Autodesk Inventor part; units mm, degrees
ref_plane "YZ Plane" through (0, 0, 0) normal (1, 0, 0) x (0, 1, 0)
ref_plane "XZ Plane" through (0, 0, 0) normal (0, 1, 0) x (-1, 0, 0)
ref_plane "XY Plane" through (0, 0, 0) normal (0, 0, 1) x (1, 0, 0)
sketch "Boceto1" plane through (0, 0, 0) normal (0, 0, 1) x (1, 0, 0)
  line L0 (254.0457, 0) -> (177.0228, 110)
  line L1 (77.0228, 110) -> (0, 0)
  line L2 (84.5228, 110) -> (84.5228, 55)
  line L3 (84.5228, 55) -> (96.5228, 55)
  line L4 (96.5228, 55) -> (96.5228, 110)
  line L5 (157.5228, 110) -> (157.5228, 55)
  line L6 (157.5228, 55) -> (169.5228, 55)
  line L7 (169.5228, 55) -> (169.5228, 110)
  line L8 (84.5228, 110) -> (77.0228, 110)
  line L9 (177.0228, 110) -> (169.5228, 110)
  line L10 (157.5228, 110) -> (96.5228, 110)
  line L11 (0, 0) -> (40.0401, 0)
  line L12 (40.0401, 0) -> (254.0457, 0)
  dimension "d1" = 100
  dimension "d2" = 110
  dimension "d3" = 61
  dimension "d5" = 12
  dimension "d6" = 7.5
  dimension "d12" = 55
  dimension "d23" = 55
  dimension "d24" = 55
extrude "Extrusión1" add sketch "Boceto1" along normal blind 6
sketch "Boceto3" plane through (0, 0, 6) normal (0, 0, 1) x (1, 0, 0)
  line L0 (0, 0) -> (254.0457, 0)
  line L1 (50, 9) -> (50, 0)
  line L2 (45, 0) -> (45, 9)
  line L3 (43.5, 12) -> (51.5, 12)
  line L4 (51.5, 12) -> (51.5, 9)
  line L5 (43.5, 9) -> (43.5, 12)
  line L6 (51.5, 9) -> (50, 9)
  line L7 (45, 9) -> (43.5, 9)
  line L8 (157.5228, 110) -> (96.5228, 110)
  line L9 (127.0228, 110) -> (127.0228, 0)
  line L10 (204.0457, 9) -> (204.0457, 0)
  line L11 (209.0457, 0) -> (209.0457, 9)
  line L12 (210.5457, 12) -> (202.5457, 12)
  line L13 (202.5457, 12) -> (202.5457, 9)
  line L14 (210.5457, 9) -> (210.5457, 12)
  line L15 (202.5457, 9) -> (204.0457, 9)
  line L16 (209.0457, 9) -> (210.5457, 9)
  line L17 (45, 0) -> (50, 0) construction
  line L18 (204.0457, 0) -> (209.0457, 0) construction
  point P0 (204.0457, 0)
  point P1 (47.5, 12)
  point P2 (47.5, 0)
  point P3 (206.5457, 0)
  dimension "d25" = 5
  dimension "d26" = 8
  dimension "d27" = 12
  dimension "d29" = 45
  dimension "d30" = 3
extrude "Extrusión3" cut sketch "Boceto3" against normal up to next
sketch "Boceto4" plane through (0, 0, 0) normal (0, -1, 0) x (1, 0, 0)
  line L0 (77.0228, 6) -> (0, 6)
  line L1 (77.0228, 0) -> (0, 0)
  line L2 (38.5114, 6) -> (28.5114, 6)
  line L3 (28.5114, 6) -> (28.5114, 0)
  line L4 (28.5114, 0) -> (38.5114, 0)
  line L5 (38.5114, 0) -> (38.5114, 6)
  line L6 (50, 0) -> (204.0457, 0)
  line L7 (56.5114, 6) -> (66.5114, 6)
  line L8 (66.5114, 6) -> (66.5114, 0)
  line L9 (66.5114, 0) -> (56.5114, 0)
  line L10 (56.5114, 0) -> (56.5114, 6)
  line L11 (157.5228, 0) -> (96.5228, 0)
  line L12 (127.0228, 0) -> (127.0228, 6) construction
  line L13 (215.5342, 6) -> (225.5342, 6)
  line L14 (225.5342, 6) -> (225.5342, 0)
  line L15 (225.5342, 0) -> (215.5342, 0)
  line L16 (215.5342, 0) -> (215.5342, 6)
  line L17 (197.5342, 6) -> (187.5342, 6)
  line L18 (187.5342, 6) -> (187.5342, 0)
  line L19 (187.5342, 0) -> (197.5342, 0)
  line L20 (197.5342, 0) -> (197.5342, 6)
  dimension "d33" = 10
  dimension "d34" = 18
  dimension "d35" = 10
extrude "Extrusión4" add sketch "Boceto4" along normal blind 3 contours L8 L1 L10 L0 | L18 L17 L20 L6 | L5 L1 L3 L0 | L13 L14 L15 L16
sketch "Boceto5" plane through (0, 0, 6) normal (0, 0, 1) x (1, 0, 0)
  circle A0 centre (127.0228, 32) radius 2
  line L0 (66.5114, 0) -> (187.5342, 0)
  line L1 (157.5228, 110) -> (96.5228, 110)
  point P0 (0, 0)
  point P1 (127.0228, 110)
  dimension "d39" = 4
  dimension "d40" = 32
extrude "Extrusión5" cut sketch "Boceto5" against normal through all
properties part number "UnionColumnas"
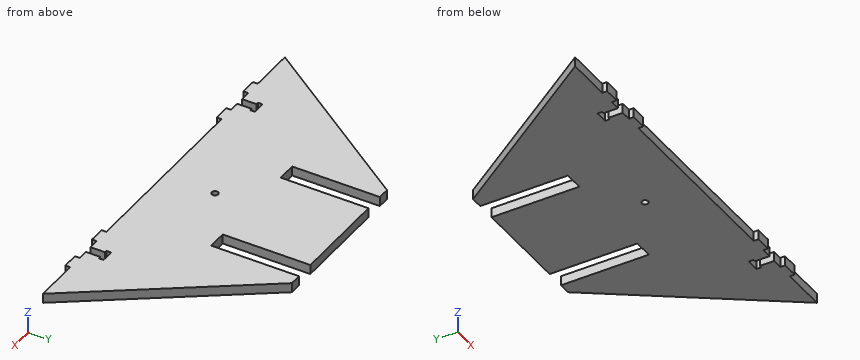
The listing builds one solid part. Answer for the finished solid, in the listing's coordinates (mm). Round coordinates to 2 decimals unless told otherwise and drop trailing zeros. Write each loop counter-clockwise with the first axis right and the second up, starting at its lowest first coordinate (ties: lowest second). Pieces come first, ordered by that corner, then holes. Notation, with made-up numbers: (23.25, 37) - (68.25, 37) arc R9 cw to (68.25, 48) - close; hole circle Ø8 at (-12, -16). An arc over 180 degrees is marked (long way). Use a Markdown table: item, result. Add a question column.
1. The part is cut by section B-B (x = 100). Write down the section's boundary in (y, z), and give its area (3 significant figures).
2. The part is cut by section D-D (x = 191.5). Write down the section's boundary in (y, z).
3. The part is cut by section C-C (y = 63.5). Write down the section's boundary in (x, z).
4. Flat-ended cylindrical pins translate along their axes: P1, Ø1.5, axis at y = -2, z = 2.5, coming from the -X side; P2, Ø2, axis at x = 139, z = 3, coming from the -Y side; P3, Ø0.8, axis at x = 203.5, z = 2.5, coming from the +Y side. Find the tip coordinate at first contact, or state that the pin passes through.
5. The part is cut by section A-A (y = 83). Write down the section's boundary in (x, z).
6. Consider line 1 (X direction, y = 58.5, z = 2.25); line 2 (X direction, y = 69.5, z = 2.1); line 3 (Y direction, x = 147.5, z = 5.7). Determine where each line is inside the solid, lowest interval first.
Reported:
| question | item | result |
|---|---|---|
| 1 | outline | (0, 0) - (110, 0) - (110, 6) - (0, 6) - close |
| 1 | area | 660 mm^2 |
| 2 | outline | (-3, 0) - (89.32, 0) - (89.32, 6) - (-3, 6) - close |
| 3 | outline | (44.46, 0) - (84.52, 0) - (84.52, 6) - (44.46, 6) - close; (96.52, 0) - (157.52, 0) - (157.52, 6) - (96.52, 6) - close; (169.52, 0) - (209.58, 0) - (209.58, 6) - (169.52, 6) - close |
| 4 | P1 | x = 28.51 |
| 4 | P2 | y = 0 |
| 4 | P3 | y = 72.76 |
| 5 | outline | (58.12, 0) - (84.52, 0) - (84.52, 6) - (58.12, 6) - close; (96.52, 0) - (157.52, 0) - (157.52, 6) - (96.52, 6) - close; (169.52, 0) - (195.93, 0) - (195.93, 6) - (169.52, 6) - close |
| 6 | line 1 | 40.96 to 84.52, 96.52 to 157.52, 169.52 to 213.08 |
| 6 | line 2 | 48.66 to 84.52, 96.52 to 157.52, 169.52 to 205.38 |
| 6 | line 3 | 0 to 110 |
